Read the model definition and answer for the solid it produces. Units are mm, in the model's axes. A direction names the side the tool comes from. Coordinates: 2 decimals unless noted, no trailing zeros. Put each result on its own line as item: value.
from build123d import *

# Parameters (mm, degrees)
SKETCH_2_OUTSIDE_W  = 123.846
SKETCH_2_OUTSIDE_H  = 123.846
SKETCH_2_OUTSIDE_R  = 17
CUT_EXTRUDE_1_DEPTH = 2
SKETCH_3_OUTSIDE_W  = 123.846
SKETCH_3_OUTSIDE_H  = 123.846
SKETCH_3_OUTSIDE_R  = 22
CUT_EXTRUDE_2_DEPTH = 2
CUT_EXTRUDE_3_DEPTH = 107.609099049
CHAMFER_1_SIZE      = 2.5


with BuildPart() as part:
    # 草图1 → 旋转1 (revolve)
    with BuildSketch(Plane(origin=(0, 0, 0), x_dir=(0, 0, -1), z_dir=(1, 0, 0)), mode=Mode.PRIVATE) as revolve_1_sk:
        Polygon((0, 0), (0, 17.5), (17, 17.5), (17, 21.5), (37, 21.5), (37, 22.5), (62, 22.5), (62, 30), (64, 30), (64, 45.5), (68.796097738, 45.5), (85, 13), (85, 0), align=None)
    revolve(revolve_1_sk.sketch.rotate(Axis((0, 0, -85), (0, 0, 1)), 90), axis=Axis((0, 0, -85), (0, 0, 1)))

    # 草图2 outside → 切除-拉伸1 (cut)
    with BuildSketch(Plane.XY.offset(-17)):
        Rectangle(SKETCH_2_OUTSIDE_W, SKETCH_2_OUTSIDE_H)
        Circle(SKETCH_2_OUTSIDE_R, mode=Mode.SUBTRACT)
    extrude(amount=CUT_EXTRUDE_1_DEPTH, mode=Mode.SUBTRACT)

    # 草图3 outside → 切除-拉伸2 (cut)
    with BuildSketch(Plane.XY.offset(-62)):
        Rectangle(SKETCH_3_OUTSIDE_W, SKETCH_3_OUTSIDE_H)
        Circle(SKETCH_3_OUTSIDE_R, mode=Mode.SUBTRACT)
    extrude(amount=CUT_EXTRUDE_2_DEPTH, mode=Mode.SUBTRACT)

    # 草图4 → 切除-拉伸3 (cut, through all)
    with BuildSketch(Plane.XY):
        with BuildLine():
            Line((-3, 10.062305899), (-3, 7.416198487))
            ThreePointArc((-3, 7.416198487), (-5.656854249, 5.656854249), (-7.416198487, 3))
            Line((-7.416198487, 3), (-10.062305899, 3))
            ThreePointArc((-10.062305899, 3), (-10.5, 0), (-10.062305899, -3))
            Line((-10.062305899, -3), (-7.416198487, -3))
            ThreePointArc((-7.416198487, -3), (-5.656854249, -5.656854249), (-3, -7.416198487))
            Line((-3, -7.416198487), (-3, -10.062305899))
            ThreePointArc((-3, -10.062305899), (0, -10.5), (3, -10.062305899))
            Line((3, -10.062305899), (3, -7.416198487))
            ThreePointArc((3, -7.416198487), (5.656854249, -5.656854249), (7.416198487, -3))
            Line((7.416198487, -3), (10.062305899, -3))
            ThreePointArc((10.062305899, -3), (10.5, 0), (10.062305899, 3))
            Line((10.062305899, 3), (7.416198487, 3))
            ThreePointArc((7.416198487, 3), (5.656854249, 5.656854249), (3, 7.416198487))
            Line((3, 7.416198487), (3, 10.062305899))
            ThreePointArc((3, 10.062305899), (0, 10.5), (-3, 10.062305899))
        make_face()
    extrude(amount=-CUT_EXTRUDE_3_DEPTH, mode=Mode.SUBTRACT)

    # 倒角1
    chamfer_1_edges = [part.edges().sort_by_distance(p)[0] for p in [
        (5.656854249, -5.656854249, -85),
        (5.656854249, 5.656854249, -85),
        (-5.656854249, 5.656854249, -85),
        (-5.656854249, -5.656854249, -85),
        (-5.656854249, -5.656854249, 0),
        (5.656854249, -5.656854249, 0),
        (5.656854249, 5.656854249, 0),
        (-5.656854249, 5.656854249, 0),
    ]]
    chamfer(chamfer_1_edges, length=CHAMFER_1_SIZE)


solid = part.part
1) Which of the six approach directions +Z, -Z, +X, -X, +Y, -Y give full straight-line access (tool end or side, diameter ignored) to faces 1 (the flat face through (8, 8, 0)), 2 (the cylindrical face through (5.689, 5.625, -41.94))?
Answer list:
face 1: +Z, +X, -X, +Y, -Y
face 2: +Z, -Z
2) Straight lines are drawn through the part: line 1 (X direction, y = -2.5, z = -44); line 2 (Y direction, x = -6, z = -76); line 3 (X direction, y = -4.5, z = -68.5). For each, find the intervals that lie inside material, in ascending order. Write a range as [from, to].
Answer list:
line 1: x = [-22.36, -10.2], [10.2, 22.36]
line 2: y = [-30.47, -5.29], [5.29, 30.47]
line 3: x = [-45.28, -6.61], [6.61, 45.28]
3) Determine the mould class of faces 3 (the conical face through (-6.6, -6.51, -83.77)), 4 (the flat face through (22, 2, -37)), 5 (the cylindrical face through (-4.769, -21.477, -61.014)), 6 (the cylindrical face through (5.625, -5.689, -41.94)) for opening direction Z: released by +Z, released by -Z, zero draft, split by the parting line, or undercut.
Answer list:
face 3: released by -Z
face 4: released by +Z
face 5: undercut
face 6: zero draft
4) Given pin 1 Ø0.8 at (x, z) = (-9.5, -40) entering from -Y; pin 2 Ø8 at (x, y) = (-0.5, 35.5) entering from -Z; pin 3 Ø1.3 at (x, z) = (9, -22) entering from -Y, each flat-ended and moving along its own axis, determine where each tip first touches the part or whether it passes through.
Answer list:
pin 1: stops at y = -20.58
pin 2: stops at z = -75.77
pin 3: stops at y = -19.81
